Part model, mm, in its own coordinate system. Give positions to 0.01 mm unless a question says otherwise; leave off trailing zeros. Order: outer loops, then holes, each group sorted by start corner. A loop starts at its lowest first (then second) coordinate and runs counter-clockwise, first axis right, second up. Notation, with made-up numbers: (18.5, 55.25) -> (23.5, 55.25) arc R18 cw to (23.5, 69.25) -> close; hole circle Ø10 at (0.25, 89). An arc over 180 degrees is marked (long way). Write item = value, one per line. Start each with the question number.
(1) Two-plate mould, pull along X, no slides. Class faces 1 (the cylindrical face through (26, 31, 132)), 2 (the cylindrical face through (4.336, -19.524, 128.18)), 3 (the flat face through (-28, -3, 128)): pulls with the +X half, pulls with the -X half, needs draft (parallel to the pull), parting line crosses it, or undercut.
(2) Saw through at C-C, the plane z = 52.5. List the corners of the cut face in (x, y), then the cut area to 3 significant figures.
(3) Flat gauge pins, fed straight in: pin 1 (24 mm diameter, centred on x = 0, y = 0, fed in from +Z); pin 2 (12 mm diameter, centred on x = -2, y = 14.5, fed in from -Z). Where does each tip first touch, or does it go through?
(4) Probe line 1 along Y through (x, z) = (0, 105); line 2 along Y through (x, z) = (14.5, 212); line 3 along X through (y, z) = (-12, 137.5). List the from-to ranges inside material, lowest first. Write a range as from..to.
(5) Saw through at A-A, the plane x = 0. List the corners of the cut face in (y, z), then the cut area to 3 significant figures.
(6) Saw through at B-B, the plane y = 0. List the corners of the cut face in (x, z), then the cut area to 3 significant figures.
from build123d import *

# Parameters (mm, degrees)
SKETCH_8_W          = 56
SKETCH_8_H          = 64
EXTRUDE_1_DEPTH     = 260
SKETCH_9_R          = 20
CUT_EXTRUDE_1_DEPTH = 264.453980801
FILLET_1_R          = 5


with BuildPart() as part:
    # 草图8 → 凸台-拉伸1 (new body)
    with BuildSketch(Plane.XY):
        Rectangle(SKETCH_8_W, SKETCH_8_H)
    extrude(amount=EXTRUDE_1_DEPTH)

    # 草图9 → 切除-拉伸1 (cut, through all)
    with BuildSketch(Plane(origin=(0, 0, 0), x_dir=(-1, 0, 0), z_dir=(0, 0, -1))):
        Circle(SKETCH_9_R)
    extrude(amount=-CUT_EXTRUDE_1_DEPTH, mode=Mode.SUBTRACT)

    # 圆角1
    fillet_1_edges = [part.edges().sort_by_distance(p)[0] for p in [
        (-28, 32, 130),
        (28, 32, 130),
        (28, -32, 130),
    ]]
    fillet(fillet_1_edges, radius=FILLET_1_R)


solid = part.part
Results list:
q1.face_1 = pulls with the +X half
q1.face_2 = undercut
q1.face_3 = pulls with the -X half
q2.outline = (-28, -32) -> (23, -32) arc R5 ccw to (28, -27) -> (28, 27) arc R5 ccw to (23, 32) -> (-23, 32) arc R5 ccw to (-28, 27) -> close; hole circle Ø40 at (0, 0)
q2.area = 2,310 mm^2
q3.pin_1 = through
q3.pin_2 = 0
q4.line_1 = -32..-20, 20..32
q4.line_2 = -32..-13.77, 13.77..32
q4.line_3 = -28..-16, 16..28
q5.outline = (-32, 0) -> (-20, 0) -> (-20, 260) -> (-32, 260) -> close; (20, 0) -> (32, 0) -> (32, 260) -> (20, 260) -> close
q5.area = 6,240 mm^2
q6.outline = (-28, 0) -> (-20, 0) -> (-20, 260) -> (-28, 260) -> close; (20, 0) -> (28, 0) -> (28, 260) -> (20, 260) -> close
q6.area = 4,160 mm^2
